Read the model definition and answer for the solid it produces. Units are mm, in the model's axes. Face numbers are marked on the shaded views. A direction names the side the tool comes from. Give positions to 0.01 mm unless a question says otherwise; leave off trailing zeros. Loops run counter-clockwise (first coordinate to the right, second up) from the corner with the lowest first, then second, coordinate; pieces in that order, holes last. Notation, with made-up numbers: (72.5, -15) -> (81.5, -15) arc R20 cw to (81.5, 17) -> close; hole circle Ø4 at (-4.5, -1.75). An arc over 180 degrees is marked (long way). Write each question's results on one line, items separated by ' | '. Start each with the question number.
Item 1: Which of the six approach directions +Z, -Z, +X, -X, +Y, -Y give full straight-line access (tool end or side, diameter ignored) to the marked faces 1, 2, 3, 4 and 5?
Item 2: Section B-B on z = 2 is taken. Write down the section's boundary in (x, y).
Item 3: Section D-D on y = -18 is taken. Write down the section's boundary in (x, z).
Item 4: Section C-C on x = -36 is taken. Write down the section's boundary in (y, z), and give its area (3 significant figures).
Item 5: Section A-A on y = -34.5 is taken. Write down the section's boundary in (x, z), and give its area (3 significant figures).
Item 6: Find the intervals of material crossed by line 1 (Y direction, x = -28, z = -8.5); line 2 (Z direction, x = -25.5, y = -30), in increasing order.
Item 7: Each of these flat-tipped pins is pushed along its axis until it touches: P1, Ø7.5, axis at y = -38.5, z = 32.5, coming from the +X side; P2, Ø12.5, axis at y = -36.5, z = -91, coming from the -X side; P3, Ø5, axis at x = -40, y = -22.5, coming from the +Z side. Where does it stop, or does it pass through?
```python
from build123d import *

# Parameters (mm, degrees)
F0_W     = 88.8999989152
F0_H     = 165.0999989152
F1_DEPTH = 6.35
F2_DEPTH = 25.4
F3_DEPTH = 50.8
F4_R     = 5.08
F5_SIZE2 = 7.3323484187
F5_SIZE  = 12.7


with BuildPart() as f1:
    # F0 (on Front) → F1 (new body)
    with BuildSketch(Plane.XZ):
        with Locations((-9.271614182, -26.4538442612)):
            Rectangle(F0_W, F0_H)
        Polygon((-47.371614182, 11.6461557388), (-47.371614182, 49.7461557388), (-9.271614182, 49.7461557388), (28.828385818, 49.7461557388), (28.828385818, -64.5538442612), (28.828385818, -102.6538442612), (-9.271614182, -102.6538442612), (-47.371614182, -102.6538442612), align=None, mode=Mode.SUBTRACT)
    extrude(amount=F1_DEPTH)

    # F0 (on Front) → F2 (join)
    with BuildSketch(Plane.XZ):
        with BuildLine():
            Line((-21.971614182, 11.6461557388), (-47.371614182, 11.6461557388))
            Line((-47.371614182, 11.6461557388), (-47.371614182, -102.6538442612))
            Line((-47.371614182, -102.6538442612), (-9.271614182, -102.6538442612))
            Line((-9.271614182, -102.6538442612), (-9.271614182, -77.2538442612))
            ThreePointArc((-9.271614182, -77.2538442612), (-5.5518703031, -68.2735881401), (3.428385818, -64.5538442612))
            Line((3.428385818, -64.5538442612), (28.828385818, -64.5538442612))
            Line((28.828385818, -64.5538442612), (28.828385818, 49.7461557388))
            Line((28.828385818, 49.7461557388), (-9.271614182, 49.7461557388))
            Line((-9.271614182, 49.7461557388), (-9.271614182, 24.3461557388))
            ThreePointArc((-9.271614182, 24.3461557388), (-12.9913580609, 15.3658996178), (-21.971614182, 11.6461557388))
        make_face()
    extrude(amount=F2_DEPTH)

    # F0 (on Front) → F3 (join)
    with BuildSketch(Plane.XZ):
        with BuildLine():
            Line((-9.271614182, 49.7461557388), (-47.371614182, 49.7461557388))
            Line((-47.371614182, 49.7461557388), (-47.371614182, 11.6461557388))
            Line((-47.371614182, 11.6461557388), (-21.971614182, 11.6461557388))
            ThreePointArc((-21.971614182, 11.6461557388), (-12.9913580609, 15.3658996178), (-9.271614182, 24.3461557388))
            Line((-9.271614182, 24.3461557388), (-9.271614182, 49.7461557388))
        make_face()
        with BuildLine():
            Line((-9.271614182, -77.2538442612), (-9.271614182, -102.6538442612))
            Line((-9.271614182, -102.6538442612), (28.828385818, -102.6538442612))
            Line((28.828385818, -102.6538442612), (28.828385818, -64.5538442612))
            Line((28.828385818, -64.5538442612), (3.428385818, -64.5538442612))
            ThreePointArc((3.428385818, -64.5538442612), (-5.5518703031, -68.2735881401), (-9.271614182, -77.2538442612))
        make_face()
    extrude(amount=F3_DEPTH)

    # F4
    f4_edges = [f1.edges().sort_by_distance(p)[0] for p in [
        (35.178385, -6.35, -26.453844),
        (-9.271614, -6.35, -109.003844),
        (-53.721614, -6.35, -26.453844),
        (-9.271614, -6.35, 56.096155),
    ]]
    fillet(f4_edges, radius=F4_R)

    # F5
    f5_edges = [f1.edges().sort_by_distance(p)[0] for p in [
        (-47.371614, -50.8, 30.696156),
        (-28.321614, -50.8, 49.746156),
        (9.778386, -50.8, -102.653844),
        (28.828386, -50.8, -83.603844),
        (28.828386, -25.4, -7.403844),
        (-47.371614, -25.4, -45.503844),
        (-28.321614, -25.4, -102.653844),
        (9.778386, -25.4, 49.746156),
    ]]
    chamfer(f5_edges, length=F5_SIZE, length2=F5_SIZE2)


solid = f1.part
```
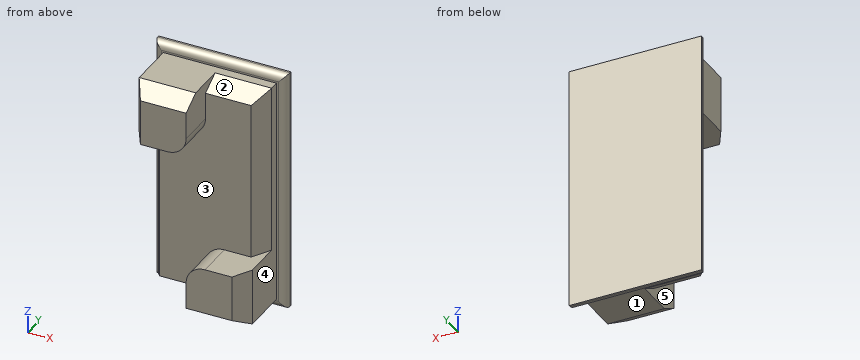
Findings:
1) face 1: -Z, +X, -X, -Y | face 2: +Z, +X, -Y | face 3: -Y | face 4: +Z, -Z, +X, -Y | face 5: -Z, -X, -Y
2) outline: (-53.72, -1.27) arc R5.08 ccw to (-48.64, -6.35) -> (-47.37, -6.35) -> (-47.37, -12.7) -> (-40.04, -25.4) -> (21.5, -25.4) -> (28.83, -12.7) -> (28.83, -6.35) -> (30.1, -6.35) arc R5.08 ccw to (35.18, -1.27) -> (35.18, 0) -> (-53.72, 0) -> close
3) outline: (-47.37, 11.65) -> (-44.31, 11.65) -> (-44.31, -99.59) -> (-9.27, -99.59) -> (-9.27, -102.65) -> (28.83, -102.65) -> (28.83, -64.55) -> (25.77, -64.55) -> (25.77, 46.69) -> (-9.27, 46.69) -> (-9.27, 49.75) -> (-47.37, 49.75) -> close
4) outline: (-50.8, 11.65) -> (-25.4, 11.65) -> (-25.4, -95.32) -> (-12.7, -102.65) -> (-6.35, -102.65) -> (-6.35, -103.92) arc R5.08 ccw to (-1.27, -109) -> (0, -109) -> (0, 56.1) -> (-1.27, 56.1) arc R5.08 ccw to (-6.35, 51.02) -> (-6.35, 49.75) -> (-38.1, 49.75) -> (-50.8, 42.41) -> close | area: 4,820 mm2
5) outline: (-47.37, 11.65) -> (-21.97, 11.65) arc R12.7 ccw to (-9.27, 24.35) -> (-9.27, 49.75) -> (-47.37, 49.75) -> close; (-9.27, -102.65) -> (28.83, -102.65) -> (28.83, -64.55) -> (3.43, -64.55) arc R12.7 ccw to (-9.27, -77.25) -> close | area: 2,830 mm2
6) line 1: -25.4 to 0 | line 2: 11.65 to 49.75
7) P1: x = -9.27 | P2: x = -9.27 | P3: z = 49.75
